```python
from build123d import *

# Parameters (mm, degrees)
F0_W     = 1
F0_H     = 5.5
F0_H_2   = 1
F0_W_2   = 5.5
F1_DEPTH = 93.07
F3_DEPTH = 12
F4_R     = 8.29
F5_DEPTH = 1
F6_DEPTH = 1.2
F7_DEPTH = 1.2


with BuildPart() as f1:
    # F0 (on Right) → F1 (new body)
    with BuildSketch(Plane.YZ):
        with Locations((0, 3.25)):
            Rectangle(F0_W, F0_H)
        Rectangle(F0_W, F0_H_2)
        with Locations((3.25, 0)):
            Rectangle(F0_W_2, F0_H_2)
        with Locations((-3.25, 0)):
            Rectangle(F0_W_2, F0_H_2)
        with Locations((0, -3.25)):
            Rectangle(F0_W, F0_H)
    extrude(amount=F1_DEPTH)

    # F2 (on face) → F3 (join)
    with BuildSketch(Plane.YZ.offset(93.07)):
        with BuildLine():
            ThreePointArc((-6, -0.5), (-4.2573465915, -4.2573465915), (-0.5, -6))
            Line((-0.5, -6), (-0.5, -0.5))
            Line((-0.5, -0.5), (-6, -0.5))
        make_face()
        with BuildLine():
            ThreePointArc((0.5, -6), (4.2573465915, -4.2573465915), (6, -0.5))
            Line((6, -0.5), (0.5, -0.5))
            Line((0.5, -0.5), (0.5, -6))
        make_face()
        Polygon((6, -0.5), (6, 0.5), (0.5, 0.5), (0.5, 6), (-0.5, 6), (-0.5, 0.5), (-6, 0.5), (-6, -0.5), (-0.5, -0.5), (-0.5, -6), (0.5, -6), (0.5, -0.5), align=None)
        with BuildLine():
            Line((-0.5, 0.5), (-0.5, 6))
            ThreePointArc((-0.5, 6), (-4.2573465915, 4.2573465915), (-6, 0.5))
            Line((-6, 0.5), (-0.5, 0.5))
        make_face()
        with BuildLine():
            Line((0.5, 0.5), (6, 0.5))
            ThreePointArc((6, 0.5), (4.2573465915, 4.2573465915), (0.5, 6))
            Line((0.5, 6), (0.5, 0.5))
        make_face()
    extrude(amount=F3_DEPTH)

    # F4 (on face) → F5 (join)
    with BuildSketch(Plane(origin=(0, 0, 0), x_dir=(0, -1, 0), z_dir=(-1, 0, 0))):
        Circle(F4_R)
        Polygon((-0.5, 6), (0.5, 6), (0.5, 0.5), (6, 0.5), (6, -0.5), (0.5, -0.5), (0.5, -6), (-0.5, -6), (-0.5, -0.5), (-6, -0.5), (-6, 0.5), (-0.5, 0.5), align=None, mode=Mode.SUBTRACT)
        Polygon((0.5, 0.5), (0.5, 6), (-0.5, 6), (-0.5, 0.5), (-6, 0.5), (-6, -0.5), (-0.5, -0.5), (-0.5, -6), (0.5, -6), (0.5, -0.5), (6, -0.5), (6, 0.5), align=None)
    extrude(amount=F5_DEPTH)

    # F4 (on face) → F6 (join)
    with BuildSketch(Plane(origin=(0, 0, 0), x_dir=(0, -1, 0), z_dir=(-1, 0, 0))):
        Circle(F4_R)
        Polygon((-0.5, 6), (0.5, 6), (0.5, 0.5), (6, 0.5), (6, -0.5), (0.5, -0.5), (0.5, -6), (-0.5, -6), (-0.5, -0.5), (-6, -0.5), (-6, 0.5), (-0.5, 0.5), align=None, mode=Mode.SUBTRACT)
    extrude(amount=F6_DEPTH)

    # F4 (on face) → F7 (join)
    with BuildSketch(Plane(origin=(0, 0, 0), x_dir=(0, -1, 0), z_dir=(-1, 0, 0))):
        Polygon((0.5, 0.5), (0.5, 6), (-0.5, 6), (-0.5, 0.5), (-6, 0.5), (-6, -0.5), (-0.5, -0.5), (-0.5, -6), (0.5, -6), (0.5, -0.5), (6, -0.5), (6, 0.5), align=None)
    extrude(amount=F7_DEPTH)


solid = f1.part
```
Check sheet for the modelled part. Datum: model origin and axes. Units: mm. A direction names the side the tool comes from. Coordinates: 2 decimals unless noted, no trailing zeros. Order: outer loops, then holes, each group sorted by start corner. A loop starts at its lowest first (then second) coordinate and runs counter-clockwise, first axis right, second up. Notation, with made-up numbers: (-17, -17.5) -> (-13, -17.5) arc R32 cw to (-13, 9.5) -> close; hole circle Ø10 at (62.5, 35.5). An arc over 180 degrees is marked (long way). Write item = value, one per line. Start each with the question number.
1) Go/stop test with flat-tipped pins: P1, Ø0.5, axis at x = 44.5, y = 0, coming from the +Z side; P2, Ø4, axis at x = 13, z = 3.5, coming from the -Y side; P3, Ø1.6, axis at x = 43, y = 2.5, coming from the -Z side. Record where each tip stops, or that it passes through.
2) Material ranges on L1, parallel to X at y = -1, z = -4.75; L2, parallel to X at y = 6.25, z = 1.5; L3, parallel to Z at x = 66, y = -3, recorded low to high.
3) Mould release check, pull along X, two halves, no side actions. Record for faces 1 (the flat face through (-1.2, 0, 0)), 2 (the flat face through (93.07, 3, -3)), 3 (the cylindrical face through (98.986, -4.215, 4.299)): +X half, -X half, draft (parallel to the pull), parting line (faces both ways), or undercut.
4) Cross-section at B-B (y = 3.25). Enter the section's corners in (x, z), then the cut area to 3 significant figures.
5) Cross-section at A-A (x = 18). Enter the section's corners in (y, z), then the cut area to 3 significant figures.
6) Access from +Z, -Z, +X, -X, +Y, -Y to the whole of each face (thin tool, end or side, straight path). Record for faces 4 (the flat face through (0, -2, -2)), 5 (the flat face through (93.07, -3, 3)), 6 (the cylindrical face through (98.986, 4.215, -4.299)).
Ans:
q1.P1 = 6
q1.P2 = -0.5
q1.P3 = -0.5
q2.L1 = -1.2 to 0, 93.07 to 105.07
q2.L2 = -1.2 to 0
q2.L3 = -0.5 to 0.5
q3.face_1 = -X half
q3.face_2 = undercut
q3.face_3 = draft
q4.outline = (-1.2, -7.63) -> (0, -7.63) -> (0, -0.5) -> (93.07, -0.5) -> (93.07, -5.07) -> (105.07, -5.07) -> (105.07, 5.07) -> (93.07, 5.07) -> (93.07, 0.5) -> (0, 0.5) -> (0, 7.63) -> (-1.2, 7.63) -> close
q4.area = 233 mm²
q5.outline = (-6, -0.5) -> (-0.5, -0.5) -> (-0.5, -6) -> (0.5, -6) -> (0.5, -0.5) -> (6, -0.5) -> (6, 0.5) -> (0.5, 0.5) -> (0.5, 6) -> (-0.5, 6) -> (-0.5, 0.5) -> (-6, 0.5) -> close
q5.area = 23.0 mm²
q6.face_4 = none
q6.face_5 = +Z, -Y
q6.face_6 = -Z, +X, +Y
